Can you work these out from the drawing? Everything is in mm from the part's minimum corner. A direction names the side the tool comes from. Give positions to 0.01 mm unless a question says otherwise; leave off trailing zeros. Write each loop counter-clockwise with the first axis right and the second up, starting at its lowest first coordinate (ties: lowest second). Pieces come first, ordered by that corner, then holes. Notation, with made-up numbers: (44.25, 45) -> (72.25, 45) arc R23 ccw to (72.25, 62) -> close; hole circle Ø6 at (28, 71.5). An arc over 180 degrees is marked (long way). Return JSON: item names as keys, results as strings.
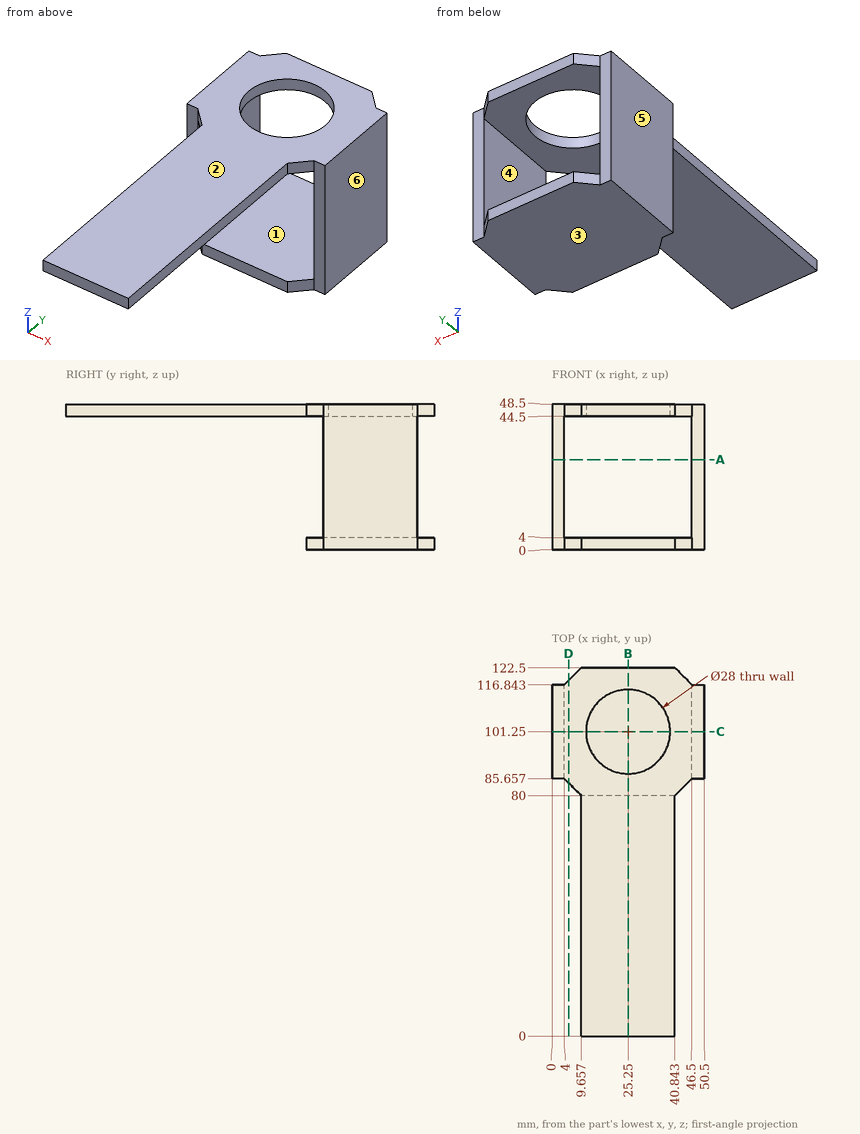
1. If I drill on line 1 (X direction, y = 111, z = 37.5); line 2 (Y direction, x = 25.25, z = 46.9); line 3 (X direction, y = 101, z = 46), over which ranges is the centre line in solid material (lowest first)? Write a range as [from, to].
Taken from the geometry:
{"line 1": "x = [0, 4], [46.5, 50.5]", "line 2": "y = [0, 87.25], [115.25, 122.5]", "line 3": "x = [0, 11.25], [39.25, 50.5]"}
2. Suppose I cut it at C-C, the plane y = 101.25. List the corners of the cut face in (x, z) for me.
Taken from the geometry:
{"outline": "(0, 0) -> (50.5, 0) -> (50.5, 48.5) -> (39.25, 48.5) -> (39.25, 44.5) -> (46.5, 44.5) -> (46.5, 4) -> (4, 4) -> (4, 44.5) -> (11.25, 44.5) -> (11.25, 48.5) -> (0, 48.5) -> close"}
3. If we mould it in two halves opening along X, with no side actions, what happens to the marked faces 3, 4, 5 and 6? For each: released by +X, released by -X, zero draft, split by the parting line, or undercut.
Taken from the geometry:
{"face 3": "zero draft", "face 4": "undercut", "face 5": "released by -X", "face 6": "released by +X"}
4. For pin 1 Ø1.2 at (x, z) = (27.5, 2) entering from -Y; pin 2 Ø2 at (x, y) = (32.5, 32.5) entering from -Z; pin 3 Ø4.5 at (x, z) = (49, 18.5) entering from -Y; pin 4 Ø4 at (x, z) = (6.5, 8) entering from -Y, each with a flat end and sliding along its axis, tell me the tip position at first contact or that it passes through.
Taken from the geometry:
{"pin 1": "stops at y = 80", "pin 2": "stops at z = 44.5", "pin 3": "stops at y = 85.66", "pin 4": "passes through"}
5. Which directions (+Z, -Z, +X, -X, +Y, -Y) give clear straight access to the entire face, cutting with the end or side of a thin tool? Please do the marked faces 1 and 2.
Taken from the geometry:
{"face 1": "+Y, -Y", "face 2": "+Z, +X, -X, +Y, -Y"}
6. Suppose I cut it at B-B, the plane x = 25.25. List the corners of the cut face in (y, z) for me.
Taken from the geometry:
{"outline": "(0, 44.5) -> (87.25, 44.5) -> (87.25, 48.5) -> (0, 48.5) -> close; (80, 0) -> (122.5, 0) -> (122.5, 4) -> (80, 4) -> close; (115.25, 44.5) -> (122.5, 44.5) -> (122.5, 48.5) -> (115.25, 48.5) -> close"}
7. Suppose I cut it at A-A, the plane z = 30. List the corners of the cut face in (x, y) for me.
Taken from the geometry:
{"outline": "(0, 85.66) -> (4, 85.66) -> (4, 116.84) -> (0, 116.84) -> close; (46.5, 85.66) -> (50.5, 85.66) -> (50.5, 116.84) -> (46.5, 116.84) -> close"}
8. Suppose I cut it at D-D, the plane x = 5.5. List the corners of the cut face in (y, z) for me.
Taken from the geometry:
{"outline": "(84.16, 0) -> (118.34, 0) -> (118.34, 4) -> (84.16, 4) -> close; (84.16, 44.5) -> (118.34, 44.5) -> (118.34, 48.5) -> (84.16, 48.5) -> close"}
